from build123d import *

# Parameters (mm, degrees)
Y_KSEKLIK_EKSTR_ZYON1_DEPTH             = 125
KES_EKSTR_ZYON1_START                   = -15
KES_EKSTR_ZYON1_DEPTH                   = 15
M3_BO_LUKLU_DELIK1_D                    = 3.2
M3_BO_LUKLU_DELIK1_DEPTH                = 11.5
M3_BO_LUKLU_DELIK1_TIP                  = 0.96137699
IZIM8_R                                 = 4
KES_EKSTR_ZYON2_DEPTH                   = 9
M3_BO_LUKLU_DELIK2_D                    = 3.2
M3_BO_LUKLU_DELIK2_DEPTH                = 11.5
M3_BO_LUKLU_DELIK2_TIP                  = 0.96137699
M3X0_5_HELISARMAL_IN_DI_LI_DELIK1_D     = 3.15
M3X0_5_HELISARMAL_IN_DI_LI_DELIK1_DEPTH = 9
M3X0_5_HELISARMAL_IN_DI_LI_DELIK1_TIP   = 0.946355475
IZIM13_R                                = 8.5
KES_EKSTR_ZYON3_DEPTH                   = 10
IZIM14_R                                = 13.5
IZIM14_R_2                              = 10.5
Y_KSEKLIK_EKSTR_ZYON2_DEPTH             = 5
RADYUS1_R                               = 1


with BuildPart() as part:
    # Çizim1 → Yükseklik-Ekstrüzyon1 (new body)
    with BuildSketch(Plane.XY):
        with BuildLine():
            ThreePointArc((-32.040014045, -45), (-33.696486936, -44.717636862), (-35.165869074, -43.902439024))
            ThreePointArc((-35.165869074, -43.902439024), (-41.1459963, -38.354523703), (-46.260809548, -32))
            Line((-46.260809548, -32), (-42.562454112, -32))
            Line((-42.562454112, -32), (-35.062454112, -32))
            Line((-35.062454112, -32), (-35.062454112, -40.077260531))
            ThreePointArc((-35.062454112, -40.077260531), (-34.622260448, -40.458146046), (-34.17792949, -40.834196891))
            ThreePointArc((-34.17792949, -40.834196891), (-32.675927184, -41.699520425), (-30.968734233, -42))
            Line((-30.968734233, -42), (30.968734233, -42))
            ThreePointArc((30.968734233, -42), (32.675927184, -41.699520425), (34.17792949, -40.834196891))
            ThreePointArc((34.17792949, -40.834196891), (34.622260448, -40.458146046), (35.062454112, -40.077260531))
            Line((35.062454112, -40.077260531), (35.062454112, -32))
            Line((35.062454112, -32), (42.562454112, -32))
            Line((42.562454112, -32), (46.260809548, -32))
            ThreePointArc((46.260809548, -32), (41.1459963, -38.354523703), (35.165869074, -43.902439024))
            ThreePointArc((35.165869074, -43.902439024), (33.696486936, -44.717636862), (32.040014045, -45))
            Line((32.040014045, -45), (-32.040014045, -45))
        make_face()
    extrude(amount=Y_KSEKLIK_EKSTR_ZYON1_DEPTH)

    # Çizim2 → Kes-Ekstrüzyon1 (cut)
    with BuildSketch(Plane.XY.offset(125).offset(KES_EKSTR_ZYON1_START)):
        with BuildLine():
            Line((30.968734233, -42), (-30.968734233, -42))
            ThreePointArc((-30.968734233, -42), (-32.675927184, -41.699520425), (-34.17792949, -40.834196891))
            ThreePointArc((-34.17792949, -40.834196891), (0, 53.25), (34.17792949, -40.834196891))
            ThreePointArc((34.17792949, -40.834196891), (32.675927184, -41.699520425), (30.968734233, -42))
        make_face()
    extrude(amount=KES_EKSTR_ZYON1_DEPTH, mode=Mode.SUBTRACT)

    # M3 Boşluklu Delik1
    with Locations(Plane(origin=(0, -45, 0), x_dir=(-1, 0, 0), z_dir=(0, -1, 0))):
        with Locations((-12.67, -117.5), (12.67, -117.5)):
            Hole(M3_BO_LUKLU_DELIK1_D / 2, depth=M3_BO_LUKLU_DELIK1_DEPTH)
            with Locations((0, 0, -(M3_BO_LUKLU_DELIK1_DEPTH + M3_BO_LUKLU_DELIK1_TIP / 2))):  # 118° drill point
                Cone(0, M3_BO_LUKLU_DELIK1_D / 2, M3_BO_LUKLU_DELIK1_TIP, mode=Mode.SUBTRACT)

    # Çizim8 → Kes-Ekstrüzyon2 (cut)
    with BuildSketch(Plane.XZ.offset(45)):
        with Locations((-41, 90)):
            Circle(IZIM8_R)
        with Locations((41, 90)):
            Circle(IZIM8_R)
        with Locations((-41, 35)):
            Circle(IZIM8_R)
        with Locations((41, 35)):
            Circle(IZIM8_R)
    extrude(amount=-KES_EKSTR_ZYON2_DEPTH, mode=Mode.SUBTRACT)

    # M3 Boşluklu Delik2
    with Locations(Plane(origin=(-41, -36, 90), x_dir=(0, 0, -1), z_dir=(0, -1, 0))):
        with Locations((0, 0), (55, 0), (0, 82), (55, 82)):
            Hole(M3_BO_LUKLU_DELIK2_D / 2, depth=M3_BO_LUKLU_DELIK2_DEPTH)
            with Locations((0, 0, -(M3_BO_LUKLU_DELIK2_DEPTH + M3_BO_LUKLU_DELIK2_TIP / 2))):  # 118° drill point
                Cone(0, M3_BO_LUKLU_DELIK2_D / 2, M3_BO_LUKLU_DELIK2_TIP, mode=Mode.SUBTRACT)

    # M3x0.5 Helisarmal İçin Dişli Delik1
    with Locations(Plane(origin=(0, 0, 0), x_dir=(-1, 0, 0), z_dir=(0, 0, -1))):
        with Locations((38.338421514, -35.130690796), (-38.338421514, -35.130690796)):
            Hole(M3X0_5_HELISARMAL_IN_DI_LI_DELIK1_D / 2, depth=M3X0_5_HELISARMAL_IN_DI_LI_DELIK1_DEPTH)
            with Locations((0, 0, -(M3X0_5_HELISARMAL_IN_DI_LI_DELIK1_DEPTH + M3X0_5_HELISARMAL_IN_DI_LI_DELIK1_TIP / 2))):  # 118° drill point
                Cone(0, M3X0_5_HELISARMAL_IN_DI_LI_DELIK1_D / 2, M3X0_5_HELISARMAL_IN_DI_LI_DELIK1_TIP, mode=Mode.SUBTRACT)

    # Çizim13 → Kes-Ekstrüzyon3 (cut)
    with BuildSketch(Plane.XZ.offset(45)):
        with Locations(Location((0, 40, 0), (0, 0, 270))):
            Circle(IZIM13_R)
    extrude(amount=-KES_EKSTR_ZYON3_DEPTH, mode=Mode.SUBTRACT)

    # Çizim14 → Yükseklik-Ekstrüzyon2 (add)
    with BuildSketch(Plane.XZ.offset(45)):
        with Locations(Location((0, 40, 0), (0, 0, 90))):
            Circle(IZIM14_R)
        with Locations(Location((0, 40, 0), (0, 0, 270))):
            Circle(IZIM14_R_2, mode=Mode.SUBTRACT)
    extrude(amount=Y_KSEKLIK_EKSTR_ZYON2_DEPTH)

    # Radyus1
    radyus1_edges = [part.edges().sort_by_distance(p)[0] for p in [
        (0, -45, 26.5),
        (0, -50, 26.5),
        (0, -50, 50.5),
    ]]
    fillet(radyus1_edges, radius=RADYUS1_R)


solid = part.part
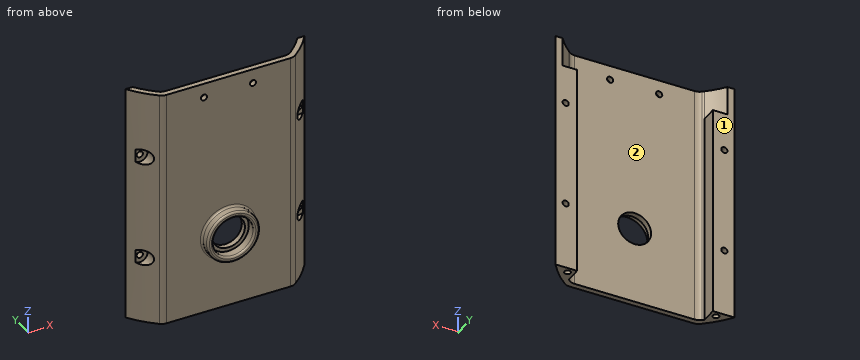
Geometry: final body of the model. Coordinates: model frame, mm. Face numbers are marked on the shaded views. A direction names the side the tool comes from. Round coordinates to 2 decimals unless told otherwise and drop trailing zeros. Loops run counter-clockwise (first coordinate to the right, second up) from the corner with the lowest first, then second, coordinate; pieces in that order, holes last. Notation, with made-up numbers: M 2,8 L 22,8 A9 ccw 22,21 Z; hole C 38,-11 d3. An arc over 180 degrees is marked long. Put each result on its own line as item: value. Start each with the question number.
(1) Section query A-A (z = 90). Return loops of the section in (x, y).
(2) Material intervals for line 1 along X through (y, z) = (-36, 108); line 2 along Z through (x, y) = (39, -37.25); line 3 along X through (y, z) = (-39, 90), sorted ascending. Write a range as [from, to].
(3) Set-up query: the marked faces 1 and 2. Return all of +Z, -Z, +X, -X, +Y, -Y with unobstructed straight access to the full face (end or side cutting, diameter ignored); none if empty.
(4) Section query C-C (x = 18.5). Return loops of the section in (y, z).
(5) Contact query for flat-ended pins moving along their axis: pin 1 Ø3 at (x, z) = (-41, 90) entering from +Y; pin 2 Ø2.5 at (y, z) = (-34.5, 34.5) entering from +X; pin 3 Ø3 at (x, z) = (-39.5, 90) entering from -Y; pin 4 Ø5 at (x, z) = (39, 90.5) entering from -Y. Output: stop coordinate, or through.
(6) Section query B-B (z = 74.5). Return loops of the section in (x, y), then the cut area to 3 significant figures.
Findings below:
1. outline: M -46.26,-32 A56.25 ccw -43.22,-36 L -42.6,-36 L -42.6,-32 Z; M -39.4,-36 L -37,-36 L -37,-42.37 A56.25 ccw -35.17,-43.9 A5 ccw -32.04,-45 L 32.04,-45 A5 ccw 35.17,-43.9 A56.25 ccw 37,-42.37 L 37,-36 L 39.4,-36 L 39.4,-32 L 35.06,-32 L 35.06,-40.08 A53.25 cw 34.18,-40.83 A5 cw 30.97,-42 L -30.97,-42 A5 cw -34.18,-40.83 A53.25 cw -35.06,-40.08 L -35.06,-32 L -39.4,-32 Z; M 42.6,-36 L 43.22,-36 A56.25 ccw 46.26,-32 L 42.6,-32 Z
2. line 1: x = [-43.22, -35.06], [35.06, 43.22]
2. line 2: z = [0, 31.54], [38.46, 86.54], [93.46, 125]
2. line 3: x = [-37, -35.06], [35.06, 37]
3. face 1: +Z, -Z, +X, -X, +Y
3. face 2: +Z, -Z, +Y
4. outline: M -45,0 L -42,0 L -42,125 L -45,125 Z
5. pin 1: passes through
5. pin 2: stops at x = 45.37
5. pin 3: stops at y = -36
5. pin 4: stops at y = -42.8
6. outline: M -46.26,-32 A56.25 ccw -35.17,-43.9 A5 ccw -32.04,-45 L 32.04,-45 A5 ccw 35.17,-43.9 A56.25 ccw 46.26,-32 L 35.06,-32 L 35.06,-40.08 A53.25 cw 34.18,-40.83 A5 cw 30.97,-42 L -30.97,-42 A5 cw -34.18,-40.83 A53.25 cw -35.06,-40.08 L -35.06,-32 Z
6. area: 361 mm2
